Part model, mm, in its own coordinate system. A direction names the side the tool comes from. Give positions to 0.01 mm unless a question says otherwise; leave off trailing zeros. Write each loop counter-clockwise with the first axis right and the second up, starting at its lowest first coordinate (ties: lowest second). Pieces come first, ordered by that corner, then holes. Notation, with made-up numbers: M 78.25,0 L 123.25,0 A33 cw 123.25,33 Z; hole C -32,25.25 d8. An arc over 180 degrees is marked long. Answer as CSV lines item,"result". Start each with the question number.
Item 1: Wall check: L1, parallel to Y at x = -28, z = 39 (3 decimals); L2, parallel to Z at x = -5.5, y = -38 (3 decimals). Give the ranges that are in metal, low to high. Write a range as from..to.
Item 2: Pin check, flat tips, straight feed: pin 1 (4 mm diameter, centred on x = -9, y = -22.5, fed in from +Z) (3 decimals); pin 2 (12 mm diameter, centred on x = -23, z = 33.5, fed in from -Y) (3 decimals). Stop position of each tip, or through.
Item 3: Band-saw the part on B-B, the plane z = 48. List the corners of the cut face in (x, y) (1 decimal).
Item 4: Band-saw the part on C-C, the plane y = -16.5. List the corners of the cut face in (x, z) (1 decimal), then the cut area to 3 significant figures.
Item 5: 3-axis set-ups, long thin cutter, end or side, ignore diameter. For faces 1 (the flat face through (-15, 0, 27)), 2 (the flat face through (-15, -26, 3.175)): which of +Z, -Z, +X, -X, +Y, -Y reach the whole face in a straight line?
Item 6: Band-saw the part on A-A, the plane x = -35. List the corners of the cut face in (y, z) (3 decimals).
from build123d import *

# Parameters (mm, degrees)
F0_W     = 45.72
F0_H     = 76.2
F1_DEPTH = 3.175
F2_W     = 45.72
F2_H     = 3.175
F3_DEPTH = 45.72
F4_W     = 45.72
F4_H     = 11.801704
F4_H_2   = 11.337079
F5_DEPTH = 25.4


with BuildPart() as f1:
    # F0 (on Front) → F1 (new body)
    with BuildSketch(Plane.XZ):
        with Locations((-14.912491, 38.1)):
            Rectangle(F0_W, F0_H)
    extrude(amount=F1_DEPTH)

    # F2 (on face) → F3 (join)
    with BuildSketch(Plane.XZ.offset(3.175)):
        with Locations((-14.912491, 1.5875)):
            Rectangle(F2_W, F2_H)
    extrude(amount=F3_DEPTH)

    # F4 (on face) → F5 (cut)
    with BuildSketch(Plane.XZ.offset(3.175)):
        with Locations((-14.912491, 70.299148)):
            Rectangle(F4_W, F4_H)
        with Locations((-14.912491, 58.729757)):
            Rectangle(F4_W, F4_H_2)
    extrude(amount=-F5_DEPTH, mode=Mode.SUBTRACT)


solid = f1.part
Output:
1,L1,"-3.175..0"
1,L2,"0..3.175"
2,pin 1,"z = 3.175"
2,pin 2,"y = -3.175"
3,outline,"M -37.8,-3.2 L 7.9,-3.2 L 7.9,0 L -37.8,0 Z"
4,outline,"M -37.8,0 L 7.9,0 L 7.9,3.2 L -37.8,3.2 Z"
4,area,"145 mm²"
5,face 1,"+Z, -Z, +X, -X, +Y"
5,face 2,"+Z, +X, -X, -Y"
6,outline,"M -48.895,0 L 0,0 L 0,53.061 L -3.175,53.061 L -3.175,3.175 L -48.895,3.175 Z"
